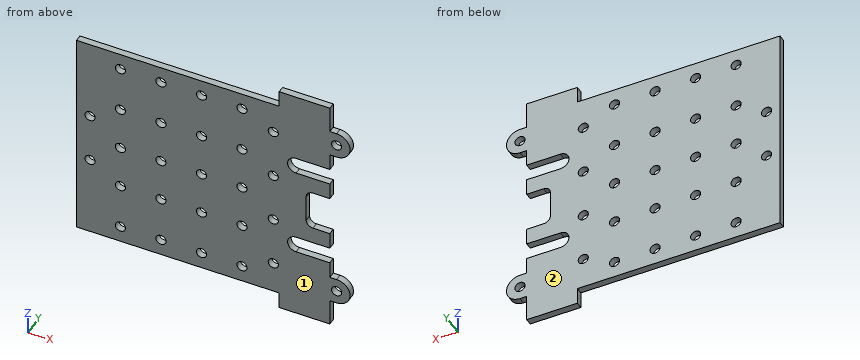
```python
from build123d import *

# Parameters (mm, degrees)
F0_R     = 1.5
F1_DEPTH = 2
F2_R     = 2


with BuildPart() as f1:
    # F0 (on Front) → F1 (new body)
    with BuildSketch(Plane.XZ):
        with BuildLine():
            Line((22.5, 16), (-37.5, 16))
            Line((-37.5, 16), (-37.5, -16))
            Line((-37.5, -16), (-26, -16))
            ThreePointArc((-26, -16), (-24.5, -14.5), (-23, -16))
            Line((-23, -16), (-14, -16))
            ThreePointArc((-14, -16), (-12.5, -14.5), (-11, -16))
            Line((-11, -16), (-2, -16))
            ThreePointArc((-2, -16), (-0.5, -14.5), (1, -16))
            Line((1, -16), (10, -16))
            ThreePointArc((10, -16), (11.5, -14.5), (13, -16))
            Line((13, -16), (30.5, -16))
            Line((30.5, -16), (30.5, -10))
            Line((30.5, -10), (37.5, -10))
            Line((37.5, -10), (37.5, -5))
            Line((37.5, -5), (27.5, -5))
            ThreePointArc((27.5, -5), (25, -2.5), (27.5, 0))
            Line((27.5, 0), (37.5, 0))
            Line((37.5, 0), (37.5, 5))
            Line((37.5, 5), (39.5, 5))
            ThreePointArc((39.5, 5), (43.5, 9), (39.5, 13))
            Line((39.5, 13), (37.5, 13))
            Line((37.5, 13), (37.5, 16))
            Line((37.5, 16), (37.5, 21))
            Line((37.5, 21), (22.5, 21))
            Line((22.5, 21), (22.5, 16))
        make_face()
        with Locations((-33.5, -8.5)):
            Circle(F0_R, mode=Mode.SUBTRACT)
        with Locations((-24.5, -2.9)):
            Circle(F0_R, mode=Mode.SUBTRACT)
        with Locations((-12.5, -2.9)):
            Circle(F0_R, mode=Mode.SUBTRACT)
        with Locations((-0.5, -2.9)):
            Circle(F0_R, mode=Mode.SUBTRACT)
        with Locations((-24.5, 11)):
            Circle(F0_R, mode=Mode.SUBTRACT)
        with Locations((-12.5, 11)):
            Circle(F0_R, mode=Mode.SUBTRACT)
        with Locations((-0.5, 11)):
            Circle(F0_R, mode=Mode.SUBTRACT)
        with Locations((20.758312, -8.5)):
            Circle(F0_R, mode=Mode.SUBTRACT)
        with Locations((11.5, -2.9)):
            Circle(F0_R, mode=Mode.SUBTRACT)
        with Locations((11.5, 11)):
            Circle(F0_R, mode=Mode.SUBTRACT)
        with Locations((20.758312, 6.5)):
            Circle(F0_R, mode=Mode.SUBTRACT)
        with Locations((39.5, 9)):
            Circle(F0_R, mode=Mode.SUBTRACT)
        with BuildLine():
            Line((-26, -16), (-37.5, -16))
            Line((-37.5, -16), (-37.5, -48))
            Line((-37.5, -48), (22.5, -48))
            Line((22.5, -48), (22.5, -53))
            Line((22.5, -53), (37.5, -53))
            Line((37.5, -53), (37.5, -48))
            Line((37.5, -48), (37.5, -45))
            Line((37.5, -45), (39.5, -45))
            ThreePointArc((39.5, -45), (43.5, -41), (39.5, -37))
            Line((39.5, -37), (37.5, -37))
            Line((37.5, -37), (37.5, -32))
            Line((37.5, -32), (27.5, -32))
            ThreePointArc((27.5, -32), (25, -29.5), (27.5, -27))
            Line((27.5, -27), (37.5, -27))
            Line((37.5, -27), (37.5, -22))
            Line((37.5, -22), (30.5, -22))
            Line((30.5, -22), (30.5, -16))
            Line((30.5, -16), (13, -16))
            ThreePointArc((13, -16), (11.5, -17.5), (10, -16))
            Line((10, -16), (1, -16))
            ThreePointArc((1, -16), (-0.5, -17.5), (-2, -16))
            Line((-2, -16), (-11, -16))
            ThreePointArc((-11, -16), (-12.5, -17.5), (-14, -16))
            Line((-14, -16), (-23, -16))
            ThreePointArc((-23, -16), (-24.5, -17.5), (-26, -16))
        make_face()
        with Locations((-24.5, -43)):
            Circle(F0_R, mode=Mode.SUBTRACT)
        with Locations((-12.5, -43)):
            Circle(F0_R, mode=Mode.SUBTRACT)
        with Locations((-0.5, -43)):
            Circle(F0_R, mode=Mode.SUBTRACT)
        with Locations((-24.5, -29.1)):
            Circle(F0_R, mode=Mode.SUBTRACT)
        with Locations((-33.5, -23.5)):
            Circle(F0_R, mode=Mode.SUBTRACT)
        with Locations((-12.5, -29.1)):
            Circle(F0_R, mode=Mode.SUBTRACT)
        with Locations((-0.5, -29.1)):
            Circle(F0_R, mode=Mode.SUBTRACT)
        with Locations((11.5, -43)):
            Circle(F0_R, mode=Mode.SUBTRACT)
        with Locations((20.758312, -38.5)):
            Circle(F0_R, mode=Mode.SUBTRACT)
        with Locations((39.5, -41)):
            Circle(F0_R, mode=Mode.SUBTRACT)
        with Locations((11.5, -29.1)):
            Circle(F0_R, mode=Mode.SUBTRACT)
        with Locations((20.758312, -23.5)):
            Circle(F0_R, mode=Mode.SUBTRACT)
    extrude(amount=F1_DEPTH)

    # F2
    f2_edges = [f1.edges().sort_by_distance(p)[0] for p in [
        (30.5, -1, -22),
        (30.5, -1, -10),
    ]]
    fillet(f2_edges, radius=F2_R)


solid = f1.part
```
Geometry check sheet. Reference: the model listing, model coordinates, mm. Face numbers are marked on the shaded views. Give positions to 0.01 mm unless a question says otherwise; leave off trailing zeros. Write each loop counter-clockwise with the first axis right and the second up, starting at its lowest first coordinate (ties: lowest second). Pieces come first, ordered by that corner, then holes. Notation, with made-up numbers: (47.5, 19) - (80.5, 19) arc R15 cw to (80.5, 48) - close; hole circle Ø3 at (52.25, 72). An arc over 180 degrees is marked (long way). Use a Markdown table: item, result.
Q1. Section check B-B, the plane x = -33.5. Enter the section's corners in (y, z).
Computed:
| item | result |
|---|---|
| outline | (-2, -48) - (0, -48) - (0, -25) - (-2, -25) - close; (-2, -22) - (0, -22) - (0, -10) - (-2, -10) - close; (-2, -7) - (0, -7) - (0, 16) - (-2, 16) - close |
Q2. Section check C-C, the plane z = -2.9. Enter the section's corners in (x, y).
Computed:
| item | result |
|---|---|
| outline | (-37.5, -2) - (-26, -2) - (-26, 0) - (-37.5, 0) - close; (-23, -2) - (-14, -2) - (-14, 0) - (-23, 0) - close; (-11, -2) - (-2, -2) - (-2, 0) - (-11, 0) - close; (1, -2) - (10, -2) - (10, 0) - (1, 0) - close; (13, -2) - (25.03, -2) - (25.03, 0) - (13, 0) - close |
Q3. Section check D-D, the plane y = -0.4. Give the number of separate pieces and of enclosed holes in the cut face, then the cut area to 3 significant figures.
Computed:
| item | result |
|---|---|
| separate pieces | 1 |
| enclosed holes | 28 |
| area | 4,630 mm² |
Q4. Section check A-A, the plane x = 36.5. Enter the section's corners in (y, z), then the cut area to 3 significant figures.
Computed:
| item | result |
|---|---|
| outline | (-2, -53) - (0, -53) - (0, -32) - (-2, -32) - close; (-2, -27) - (0, -27) - (0, -22) - (-2, -22) - close; (-2, -10) - (0, -10) - (0, -5) - (-2, -5) - close; (-2, 0) - (0, 0) - (0, 21) - (-2, 21) - close |
| area | 104 mm² |
Q5. Thickness scan on L1, parallel to Z at x = 33, y = -1.4; L2, parallel to X at y = -0.75, z = -16; L3, parallel to Z at x = 11.5, y = -0.15. Record the ranges inside material, lowest first. Write a range as [from, to].
Computed:
| item | result |
|---|---|
| L1 | z = [-53, -32], [-27, -22], [-10, -5], [0, 21] |
| L2 | x = [-37.5, -26], [-23, -14], [-11, -2], [1, 10], [13, 30.5] |
| L3 | z = [-48, -44.5], [-41.5, -30.6], [-27.6, -17.5], [-14.5, -4.4], [-1.4, 9.5], [12.5, 16] |
Q6. Go/stop test with flat-tipped pins: P1, Ø1, axis at x = 0, y = -1, coming from the -Z side; P2, Ø0.6, axis at x = 38.5, y = -1, coming from the -Z side; P3, Ø1, axis at y = -0.5, z = -3.5, coming from the +X side. Record where each tip stops, or that it passes through.
Computed:
| item | result |
|---|---|
| P1 | stops at z = -48 |
| P2 | stops at z = -45 |
| P3 | stops at x = 25.5 |
Q7. Draft check along Y on the marked faces 1 and 2. Enter one of: pulls with the +Y half, pulls with the -Y half, needs draft (parallel to the pull), parting line crosses it, or undercut.
Computed:
| item | result |
|---|---|
| face 1 | pulls with the -Y half |
| face 2 | pulls with the +Y half |
